from build123d import *

# Parameters (mm, degrees)
F0_W     = 20
F0_H     = 3
F0_R     = 12.5
F1_DEPTH = 1.5


with BuildPart() as f1:
    # F0 (on Front) → F1 (new body, symmetric)
    with BuildSketch(Plane.XZ):
        Polygon((30, 22.1), (21.5, 37.1), (-21.5, 37.1), (-30, 22.1), (-40, 22.1), (-40, 12.1), (-27, 12.1), (-27, 3.1), (-37, 3.1), (-37, -25.9), (-34, -25.9), (-27.7626620175, -53.9680209211), (-13.9565678727, -67.9), (13.9565678727, -67.9), (27.7626620175, -53.9680209211), (34, -25.9), (37, -25.9), (37, 3.1), (27, 3.1), (27, 12.1), (40, 12.1), (40, 22.1), align=None)
        with Locations((0, -35.9)):
            Rectangle(F0_W, F0_H, mode=Mode.SUBTRACT)
        with Locations((0, -6.77)):
            Circle(F0_R, mode=Mode.SUBTRACT)
    extrude(amount=F1_DEPTH, both=True)


solid = f1.part
Geometry check sheet. Reference: the model listing, model coordinates, mm. A direction names the side the tool comes from. Give positions to 0.01 mm unless a question says otherwise; leave off trailing zeros. Order: outer loops, then holes, each group sorted by start corner. A loop starts at its lowest first (then second) coordinate and runs counter-clockwise, first axis right, second up.
1) Cross-section at B-B (x = 0). Record the boundary of the cut face in (y, z), then the cut area to 3 significant figures.
Results are:
outline: (-1.5, -67.9) - (1.5, -67.9) - (1.5, -37.4) - (-1.5, -37.4) - close; (-1.5, -34.4) - (1.5, -34.4) - (1.5, -19.27) - (-1.5, -19.27) - close; (-1.5, 5.73) - (1.5, 5.73) - (1.5, 37.1) - (-1.5, 37.1) - close
area: 231 mm2
2) Cross-section at D-D (z = 30.5). Record the boundary of the cut face in (x, y).
Results are:
outline: (-25.24, -1.5) - (25.24, -1.5) - (25.24, 1.5) - (-25.24, 1.5) - close
3) Gauge pin test, flat ends, axial feed: pin 1 (0.9 mm diameter, centred on y = 0, z = -36, fed in from +X); pin 2 (0.9 mm diameter, centred on y = 0.5, z = -17, fed in from +X); pin 3 (1.5 mm diameter, centred on x = 36, y = 0, fed in from -Z). Record the tip position at first contact, or that the pin passes through.
Results are:
pin 1: stops at x = 31.86
pin 2: stops at x = 37
pin 3: stops at z = -25.9
4) Tool access check on faces 1 (the flat face through (32, 0, 3.1)), 2 (the flat face through (-35, 0, 22.1)), 3 (the flat face through (37, 0, -12)), 4 (the flat face through (-34, 0, 12.1)). Record the directions out of +Z, -Z, +X, -X, +Y, -Y that give a thin tool (end or side, any length) a straight path to the whole face; none if there is none.
Results are:
face 1: +X, +Y, -Y
face 2: +Z, -X, +Y, -Y
face 3: -Z, +X, +Y, -Y
face 4: -X, +Y, -Y
5) Material ranges on probe 1 along Z at (x, y) = (0, -0.3); probe 2 along Z at (x, y) = (5, -0.6); probe 3 along X at (y, z) = (-0.25, 9.5), recorded low to high.
Results are:
probe 1: z = -67.9 to -37.4, -34.4 to -19.27, 5.73 to 37.1
probe 2: z = -67.9 to -37.4, -34.4 to -18.23, 4.69 to 37.1
probe 3: x = -27 to 27
6) Cross-section at C-C (z = -6.77). Record the boundary of the cut face in (x, y).
Results are:
outline: (-37, -1.5) - (-12.5, -1.5) - (-12.5, 1.5) - (-37, 1.5) - close; (12.5, -1.5) - (37, -1.5) - (37, 1.5) - (12.5, 1.5) - close
7) Cross-section at A-A (y = 1.05). Record the boundary of the cut face in (x, z), then the cut area to 3 significant figures.
Results are:
outline: (-40, 12.1) - (-27, 12.1) - (-27, 3.1) - (-37, 3.1) - (-37, -25.9) - (-34, -25.9) - (-27.76, -53.97) - (-13.96, -67.9) - (13.96, -67.9) - (27.76, -53.97) - (34, -25.9) - (37, -25.9) - (37, 3.1) - (27, 3.1) - (27, 12.1) - (40, 12.1) - (40, 22.1) - (30, 22.1) - (21.5, 37.1) - (-21.5, 37.1) - (-30, 22.1) - (-40, 22.1) - close; hole circle Ø25 at (0, -6.77); hole (-10, -37.4) - (10, -37.4) - (10, -34.4) - (-10, -34.4) - close
area: 5,970 mm2
